Input: dimensioned drawing with shaded views. Units: mm. Origin: part minimum x, y, z. Coordinates: 2 decimals unless noted, no trailing zeros. Order: outer loops, then holes, each group sorted by start corner. A loop starts at its lowest first (then second) coordinate and runs counter-clockwise, first axis right, second up. Notation, with made-up numbers: (24.5, -7.75) -> (47.5, -7.75) arc R9 cw to (47.5, -2.75) -> close; hole circle Ø4 at (80.5, -24). An arc over 180 degrees is marked (long way). Write item = value, one per line. Start each with the question number.
Item 1: Mould query, pull axis X, two halves, no side actions, for the marked faces 1, 2 and 3. Classes: released by +X, released by -X, zero draft, split by the parting line, or undercut.
Item 2: Section query C-C (z = 9.25). Output: boundary loops of the cut face in (x, y) (1 decimal), then the cut area to 3 significant figures.
Item 3: Section query D-D (x = 21). Output: boundary loops of the cut face in (y, z), then the cut area to 3 significant figures.
Item 4: Section query A-A (y = 32.5). Output: boundary loops of the cut face in (x, z).
Item 5: Contact query for flat-ended pins moving along their axis: pin 1 (1 mm diameter, centred on y = 40, z = 8, fed in from -X); pin 2 (9 mm diameter, centred on x = 77.5, y = 30, fed in from +Z). Output: stop coordinate, or through.
Item 6: Ray query, line 1 along Y through (x, z) = (77.5, 5); line 2 along X through (y, z) = (32.5, 6.25); line 3 along X through (y, z) = (23.5, 12) (1 decimal). Return the intervals inside material, ascending. Write a range as [from, to].
Item 7: Section query B-B (x = 54). Output: boundary loops of the cut face in (y, z).
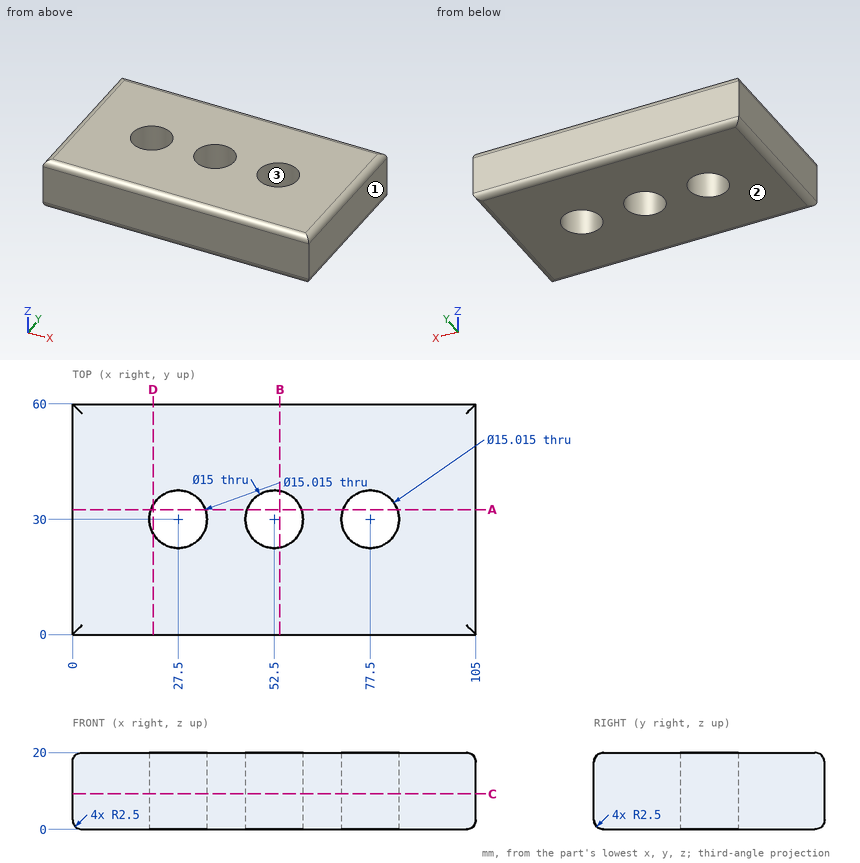
Computed:
q1.face_1 = released by +X
q1.face_2 = zero draft
q1.face_3 = undercut
q2.outline = (0, 0) -> (105, 0) -> (105, 60) -> (0, 60) -> close; hole circle Ø15 at (27.5, 30); hole circle Ø15 at (52.5, 30); hole circle Ø15 at (77.5, 30)
q2.area = 5,770 mm^2
q3.outline = (0, 2.5) arc R2.5 ccw to (2.5, 0) -> (26.24, 0) -> (26.24, 20) -> (2.5, 20) arc R2.5 ccw to (0, 17.5) -> close; (33.76, 0) -> (57.5, 0) arc R2.5 ccw to (60, 2.5) -> (60, 17.5) arc R2.5 ccw to (57.5, 20) -> (33.76, 20) -> close
q3.area = 1,040 mm^2
q4.outline = (0, 2.5) arc R2.5 ccw to (2.5, 0) -> (20.42, 0) -> (20.42, 20) -> (2.5, 20) arc R2.5 ccw to (0, 17.5) -> close; (34.58, 0) -> (45.43, 0) -> (45.43, 20) -> (34.58, 20) -> close; (59.57, 0) -> (70.42, 0) -> (70.42, 20) -> (59.57, 20) -> close; (84.58, 0) -> (102.5, 0) arc R2.5 ccw to (105, 2.5) -> (105, 17.5) arc R2.5 ccw to (102.5, 20) -> (84.58, 20) -> close
q5.pin_1 = 0
q5.pin_2 = through
q6.line_1 = [0, 22.49], [37.51, 60]
q6.line_2 = [0, 20.42], [34.58, 45.43], [59.57, 70.42], [84.58, 105]
q6.line_3 = [0, 23.7], [31.3, 48.8], [56.2, 73.7], [81.3, 105]
q7.outline = (0, 2.5) arc R2.5 ccw to (2.5, 0) -> (22.65, 0) -> (22.65, 20) -> (2.5, 20) arc R2.5 ccw to (0, 17.5) -> close; (37.35, 0) -> (57.5, 0) arc R2.5 ccw to (60, 2.5) -> (60, 17.5) arc R2.5 ccw to (57.5, 20) -> (37.35, 20) -> close
